```python
from build123d import *

# Parameters (mm, degrees)
SKETCH1_R           = 1.5875
BOSS_EXTRUDE1_DEPTH = 16.66875
CUT_EXTRUDE1_DEPTH  = 20.859618655


with BuildPart() as part:
    # Sketch1 → Boss-Extrude1 (new body)
    with BuildSketch(Plane(origin=(0, 0, 0), x_dir=(1, 0, 0), z_dir=(0, 1, 0))):
        with BuildLine():
            Line((-3.175, 0), (-3.175, 8.73125))
            Line((-3.175, 8.73125), (3.175, 8.73125))
            Line((3.175, 8.73125), (3.175, 0))
            ThreePointArc((3.175, 0), (0, -3.175), (-3.175, 0))
        make_face()
        with Locations(Location((0, 0, 0), (0, 0, 270))):
            Circle(SKETCH1_R, mode=Mode.SUBTRACT)
    extrude(amount=BOSS_EXTRUDE1_DEPTH)

    # Sketch3 → Cut-Extrude1 (cut, through all)
    with BuildSketch(Plane(origin=(3.175, 0, 0), x_dir=(0, 0, -1), z_dir=(1, 0, 0))):
        Polygon((8.73125, 13.49375), (7.14375, 13.49375), (7.14375, 15.08125), (3.175, 15.08125), (3.175, 1.5875), (7.14375, 1.5875), (7.14375, 3.175), (8.73125, 3.175), align=None)
    extrude(amount=-CUT_EXTRUDE1_DEPTH, mode=Mode.SUBTRACT)


solid = part.part
```
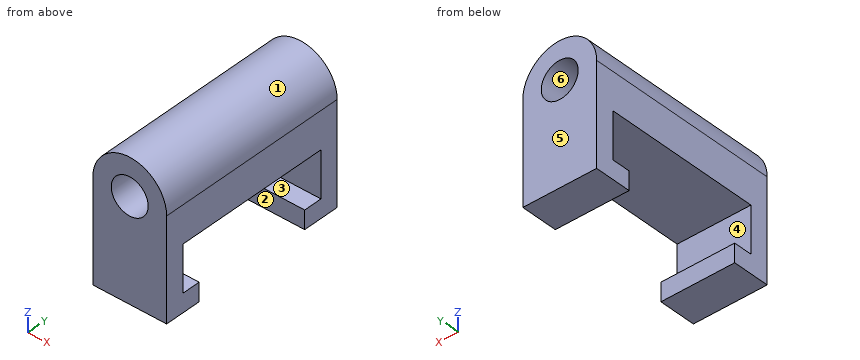
The listing builds one solid part. Answer for the finished solid, in the listing's coordinates (mm). Face numbers are marked on the shaded views. A direction names the side the tool comes from. Round coordinates to 2 decimals unless told otherwise and drop trailing zeros. Write each loop counter-clockwise with the first axis right and the second up, starting at its lowest first coordinate (ties: lowest second). Pieces come first, ordered by that corner, then holes. Notation, with made-up numbers: (60, 59.25) -> (114, 59.25) arc R27 cw to (114, 83.25) -> close; hole circle Ø3 at (7, 7.25). An arc over 180 degrees is marked (long way). Use CSV: the item, a comma, the result in double quotes. Start each with the question number.
(1) The mould has two halves that part along Y. Classify the marked faces 4, 5 and 6: released by +Y, released by -Y, zero draft, split by the parting line, or undercut.
(2) Consider L1, parallel to Y at x = -1.5, z = -8 (3 decimals); L2, parallel to Z at x = -0.5, y = 1.75 (3 decimals); L3, parallel to Y at x = -1, z = -5.75. Determine where each line is inside the solid, lowest interval first. Write a range as from..to.
(3) Which of the six approach directions +Z, -Z, +X, -X, +Y, -Y give full straight-line access (tool end or side, diameter ignored) to the marked faces 1, 2 and 3?
(4) Section C-C on x = 0 is taken. Give the vertices of the cut face in (y, z) (1 decimal), then the cut area to 3 significant figures.
(5) Section B-B on z = -7.75 is taken. Give the vertices of the cut face in (x, y) (3 decimals).
(6) Section A-A on y = 14 is taken. Count the separate pieces of the cut face and the enclosed holes in it, then the cut area to 3 significant figures.
(7) Each of these flat-tipped pins is pushed along its axis until it touches: pin 1 (3 mm diameter, centred on x = 1.5, y = 6, fed in from -Z) (3 decimals); pin 2 (1.3 mm diameter, centred on x = -1.5, y = 2, fed in from +Z); pin 3 (1.5 mm diameter, centred on x = 2.5, y = 7, fed in from +Z). Where does it stop, or does it pass through?
A:
1,face 4,"undercut"
1,face 5,"released by +Y"
1,face 6,"zero draft"
2,L1,"y = 0..3.175, 13.494..16.669"
2,L2,"z = -8.731..-7.144, -3.175..-1.507, 1.507..3.135"
2,L3,"y = 0..1.59, 15.08..16.67"
3,face 1,"+Z, +Y, -Y"
3,face 2,"-Z, +X, -X"
3,face 3,"+X, -X"
4,outline,"(0, -8.7) -> (3.2, -8.7) -> (3.2, -7.1) -> (1.6, -7.1) -> (1.6, -3.2) -> (15.1, -3.2) -> (15.1, -7.1) -> (13.5, -7.1) -> (13.5, -8.7) -> (16.7, -8.7) -> (16.7, -1.6) -> (0, -1.6) -> close; (0, 1.6) -> (16.7, 1.6) -> (16.7, 3.2) -> (0, 3.2) -> close"
4,area,"75.6 mm²"
5,outline,"(-3.175, 0) -> (3.175, 0) -> (3.175, 3.175) -> (-3.175, 3.175) -> close; (-3.175, 13.494) -> (3.175, 13.494) -> (3.175, 16.669) -> (-3.175, 16.669) -> close"
6,separate pieces,"2"
6,enclosed holes,"1"
6,area,"38.2 mm²"
7,pin 1,"stops at z = -3.175"
7,pin 2,"stops at z = 3.06"
7,pin 3,"stops at z = 2.65"
